Source: three-view drawing plus pictorial views. Frame: mm from the lowest corner of the part. Coordinates: 2 decimals unless noted, no trailing zeros. Loops run counter-clockwise (first coordinate to the right, second up) from the corner with the lowest first, then second, coordinate; pieces in that order, holes last. Notation, with made-up numbers: (72, 43) - (97, 43) arc R18 ccw to (97, 57) - close; hole circle Ø4 at (29, 3). An arc over 180 degrees is marked (long way). Return JSON: item names as keys, results as strings.
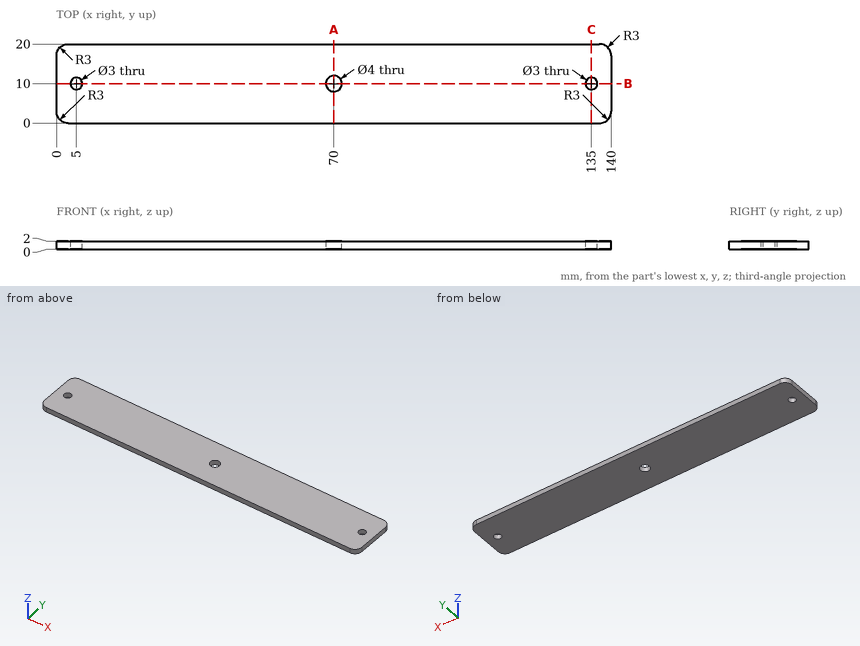
Item 1: Section query C-C, the plane x = 135. Return loops of the section in (y, z).
Worked out:
{"outline": "(0, 0) - (8.5, 0) - (8.5, 2) - (0, 2) - close; (11.5, 0) - (20, 0) - (20, 2) - (11.5, 2) - close"}
Item 2: First-contact query: pin 1 Ø3.5 at (x, y) = (135, 10) entering from -Z. Flat tip, straight axial feed; report the tip coordinate or a pass-through.
Worked out:
{"pin 1": "z = 0"}
Item 3: Section query B-B, the plane y = 10. Return loops of the section in (x, z).
Worked out:
{"outline": "(0, 0) - (3.5, 0) - (3.5, 2) - (0, 2) - close; (6.5, 0) - (68, 0) - (68, 2) - (6.5, 2) - close; (72, 0) - (133.5, 0) - (133.5, 2) - (72, 2) - close; (136.5, 0) - (140, 0) - (140, 2) - (136.5, 2) - close"}
Item 4: Section query A-A, the plane x = 70. Return loops of the section in (y, z).
Worked out:
{"outline": "(0, 0) - (8, 0) - (8, 2) - (0, 2) - close; (12, 0) - (20, 0) - (20, 2) - (12, 2) - close"}
Item 5: Ray query, probe 1 along X at (y, z) = (9.75, 1); probe 2 along Y at (x, z) = (70, 1.05); probe 3 along X at (y, z) = (10.5, 1.8). Return the intervals inside material, ascending. Write a range as from..to.
Worked out:
{"probe 1": "0..3.52, 6.48..68.02, 71.98..133.52, 136.48..140", "probe 2": "0..8, 12..20", "probe 3": "0..3.59, 6.41..68.06, 71.94..133.59, 136.41..140"}
